```python
from build123d import *

# Parameters (mm, degrees)
F0_W     = 25.4
F0_H     = 36.5125
F0_R     = 1.5875
F1_DEPTH = 1.5875
F2_W     = 19.05
F2_H     = 14.2875
F3_DEPTH = 1.5875
F4_W     = 10
F4_H     = 3.175
F5_DEPTH = 3.175


with BuildPart() as f1:
    # F0 (on Top) → F1 (new body)
    with BuildSketch(Plane.XY):
        Rectangle(F0_W, F0_H)
        with Locations((-10.715625, -16.271875)):
            Circle(F0_R, mode=Mode.SUBTRACT)
        with Locations((10.715625, -16.271875)):
            Circle(F0_R, mode=Mode.SUBTRACT)
        with Locations((-10.715625, 16.271875)):
            Circle(F0_R, mode=Mode.SUBTRACT)
        with Locations((10.715625, 16.271875)):
            Circle(F0_R, mode=Mode.SUBTRACT)
    extrude(amount=F1_DEPTH)

    # F2 (on face) → F3 (join)
    with BuildSketch(Plane.XY.offset(1.5875)):
        with Locations((0, -1.5875)):
            Rectangle(F2_W, F2_H)
    extrude(amount=F3_DEPTH)

    # F4 (on face) → F5 (join)
    with BuildSketch(Plane(origin=(0, 0, 0), x_dir=(1, 0, 0), z_dir=(0, 0, -1))):
        with Locations((0, -16.66875)):
            Rectangle(F4_W, F4_H)
    extrude(amount=F5_DEPTH)


solid = f1.part
```
CAD build for the part. Positions are in the model's coordinates, mm. A direction names the side the tool comes from. Coordinates: 2 decimals unless noted, no trailing zeros. Write each loop counter-clockwise with the first axis right and the second up, starting at its lowest first coordinate (ties: lowest second). Pieces come first, ordered by that corner, then holes.
(1) 3-axis set-ups, long thin cutter, end or side, ignore diameter. For faces 4 (the face through (0, 15.081, -2)), 5 (the face through (-5, 17, -2)), 6 (the face through (5, 17, -2)), 7 (the face through (0, -8.731, 2)): which of +Z, -Z, +X, -X, +Y, -Y reach the whole face in a straight line?
(2) Drill centre lines: probe 1 along X at (y, z) = (16, 1); probe 2 along Z at (x, y) = (5.5, 6); probe 3 along Z at (x, y) = (-7, -2) (3 decimals). Where is each one in solid material? Low to high.
(3) Cut at D-D, the plane z = 0.5. List the corners of the cut face in (x, y) (1 decimal).
(4) Cut at B-B, the plane x = 10.25. List the corners of the cut face in (y, z).
(5) Flat gauge pins, fed straight in: pin 1 (3 mm diameter, centred on x = -10.72, y = -16.27, fed in from +Z); pin 2 (1.7 mm diameter, centred on x = -2.5, z = 2.5, fed in from +Y); pin 3 (1.3 mm diameter, centred on y = -1.5, z = 3, fed in from -X) (3 decimals); pin 4 (5 mm diameter, centred on x = 10.72, y = 16.27, fed in from -Z). Where does each tip first touch, or does it go through?
(6) Two-plate mould, pull along Y, no slides. Class faces 1 (the face through (-9.525, -2, 2)), 2 (the face through (0, 5.556, 2)), 3 (the face through (12.18, 15.66, 0.78)): +Y half, -Y half, draft (parallel to the pull), parting line (faces both ways), or undercut.
(7) Cut at A-A, the plane y = 3. List the corners of the cut face in (x, z) (1 decimal).
(8) Cut at C-C, the plane x = -5.75. List the corners of the cut face in (y, z) (1 decimal).
Geometry says:
1. face 4: -Z, +X, -X, -Y
1. face 5: -Z, -X, +Y, -Y
1. face 6: -Z, +X, +Y, -Y
1. face 7: +Z, +X, -X, -Y
2. probe 1: x = -12.7 to -12.28, -9.15 to 9.15, 12.28 to 12.7
2. probe 2: z = 0 to 1.59
2. probe 3: z = 0 to 3.175
3. outline: (-12.7, -18.3) - (12.7, -18.3) - (12.7, 18.3) - (-12.7, 18.3) - close; hole circle Ø3.2 at (-10.7, -16.3); hole circle Ø3.2 at (-10.7, 16.3); hole circle Ø3.2 at (10.7, -16.3); hole circle Ø3.2 at (10.7, 16.3)
4. outline: (-18.26, 0) - (-17.79, 0) - (-17.79, 1.59) - (-18.26, 1.59) - close; (-14.75, 0) - (14.75, 0) - (14.75, 1.59) - (-14.75, 1.59) - close; (17.79, 0) - (18.26, 0) - (18.26, 1.59) - (17.79, 1.59) - close
5. pin 1: passes through
5. pin 2: stops at y = 5.56
5. pin 3: stops at x = -9.525
5. pin 4: stops at z = 0
6. face 1: draft
6. face 2: +Y half
6. face 3: undercut
7. outline: (-12.7, 0) - (12.7, 0) - (12.7, 1.6) - (9.5, 1.6) - (9.5, 3.2) - (-9.5, 3.2) - (-9.5, 1.6) - (-12.7, 1.6) - close
8. outline: (-18.3, 0) - (18.3, 0) - (18.3, 1.6) - (5.6, 1.6) - (5.6, 3.2) - (-8.7, 3.2) - (-8.7, 1.6) - (-18.3, 1.6) - close
